```python
from build123d import *

# Parameters (mm, degrees)
SKETCH1_W                                       = 98.4125
SKETCH1_H                                       = 300
BOSS_EXTRUDE1_DEPTH                             = 0.79375
CHAMFER1_SIZE                                   = 0.79375
CUT_EXTRUDE1_DEPTH                              = 2.5875
FILLET1_R                                       = 3.5
CSK_FOR_M3_FLAT_HEAD_MACHINE_SCREW1_D           = 3.4
CSK_FOR_M3_FLAT_HEAD_MACHINE_SCREW1_DEPTH       = 7.596
CSK_FOR_M3_FLAT_HEAD_MACHINE_SCREW1_CSINK_D     = 6.3
CSK_FOR_M3_FLAT_HEAD_MACHINE_SCREW1_CSINK_ANGLE = 90
CSK_FOR_M3_FLAT_HEAD_MACHINE_SCREW1_TIP         = 1.021463052


with BuildPart() as part:
    # Sketch1 → Boss-Extrude1 (new body, symmetric)
    with BuildSketch(Plane.XY):
        Rectangle(SKETCH1_W, SKETCH1_H)
    extrude(amount=BOSS_EXTRUDE1_DEPTH, both=True)

    # Chamfer1
    chamfer1_edges = [part.edges().sort_by_distance(p)[0] for p in [
        (49.20625, 0, -0.79375),
        (-49.20625, 0, -0.79375),
    ]]
    chamfer(chamfer1_edges, length=CHAMFER1_SIZE)

    # Sketch2 → Cut-Extrude1 (cut, through all)
    with BuildSketch(Plane(origin=(0, 0, -0.79375), x_dir=(-1, 0, 0), z_dir=(0, 0, -1))):
        Polygon((28.868145751, 70.95), (0, 99.818145751), (-28.868145751, 70.95), align=None)
        Polygon((-38.4125, 72.719354249), (-38.4125, 138.230645751), (-5.656854249, 105.475), align=None)
        Polygon((28.868145751, 140), (-28.868145751, 140), (0, 111.131854249), align=None)
        Polygon((38.4125, 138.230645751), (38.4125, 72.719354249), (5.656854249, 105.475), align=None)
        with BuildLine():
            Line((10, 49.95), (35, 49.95))
            ThreePointArc((35, 49.95), (38, 52.95), (35, 55.95))
            Line((35, 55.95), (10, 55.95))
            ThreePointArc((10, 55.95), (7, 52.95), (10, 49.95))
        make_face()
        with BuildLine():
            Line((-35, 21.95), (-10, 21.95))
            ThreePointArc((-10, 21.95), (-7, 24.95), (-10, 27.95))
            Line((-10, 27.95), (-35, 27.95))
            ThreePointArc((-35, 27.95), (-38, 24.95), (-35, 21.95))
        make_face()
        with BuildLine():
            Line((-35, 55.95), (-10, 55.95))
            ThreePointArc((-10, 55.95), (-7, 52.95), (-10, 49.95))
            Line((-10, 49.95), (-35, 49.95))
            ThreePointArc((-35, 49.95), (-38, 52.95), (-35, 55.95))
        make_face()
        with BuildLine():
            Line((-35, 41.95), (-10, 41.95))
            ThreePointArc((-10, 41.95), (-7, 38.95), (-10, 35.95))
            Line((-10, 35.95), (-35, 35.95))
            ThreePointArc((-35, 35.95), (-38, 38.95), (-35, 41.95))
        make_face()
        with BuildLine():
            Line((10, 41.95), (35, 41.95))
            ThreePointArc((35, 41.95), (38, 38.95), (35, 35.95))
            Line((35, 35.95), (10, 35.95))
            ThreePointArc((10, 35.95), (7, 38.95), (10, 41.95))
        make_face()
        with BuildLine():
            Line((10, 27.95), (35, 27.95))
            ThreePointArc((35, 27.95), (38, 24.95), (35, 21.95))
            Line((35, 21.95), (10, 21.95))
            ThreePointArc((10, 21.95), (7, 24.95), (10, 27.95))
        make_face()
    extrude(amount=-CUT_EXTRUDE1_DEPTH, mode=Mode.SUBTRACT)

    # Fillet1
    fillet1_edges = [part.edges().sort_by_distance(p)[0] for p in [
        (38.4125, 72.719354249, 0),
        (38.4125, 138.230645751, 0),
        (5.656854249, 105.475, 0),
        (-38.4125, 138.230645751, 0),
        (-38.4125, 72.719354249, 0),
        (-5.656854249, 105.475, 0),
        (0, 99.818145751, 0),
        (-28.868145751, 70.95, 0),
        (28.868145751, 70.95, 0),
        (28.868145751, 140, 0),
        (-28.868145751, 140, 0),
        (0, 111.131854249, 0),
    ]]
    fillet(fillet1_edges, radius=FILLET1_R)

    # CSK for M3 Flat Head Machine Screw1
    with Locations(Plane.XY.offset(0.79375)):
        with Locations((-30, -145.225), (30, -145.225), (-30, 65.7), (30, 65.7), (30, 145.225), (-30, 145.225)):
            CounterSinkHole(CSK_FOR_M3_FLAT_HEAD_MACHINE_SCREW1_D / 2, CSK_FOR_M3_FLAT_HEAD_MACHINE_SCREW1_CSINK_D / 2, depth=CSK_FOR_M3_FLAT_HEAD_MACHINE_SCREW1_DEPTH, counter_sink_angle=CSK_FOR_M3_FLAT_HEAD_MACHINE_SCREW1_CSINK_ANGLE)
            with Locations((0, 0, -(CSK_FOR_M3_FLAT_HEAD_MACHINE_SCREW1_DEPTH + CSK_FOR_M3_FLAT_HEAD_MACHINE_SCREW1_TIP / 2))):  # 118° drill point
                Cone(0, CSK_FOR_M3_FLAT_HEAD_MACHINE_SCREW1_D / 2, CSK_FOR_M3_FLAT_HEAD_MACHINE_SCREW1_TIP, mode=Mode.SUBTRACT)


solid = part.part
```
CAD build for the part. Positions are in the model's coordinates, mm. A direction names the side the tool comes from. Coordinates: 2 decimals unless noted, no trailing zeros. Write each loop counter-clockwise with the first axis right and the second up, starting at its lowest first coordinate (ties: lowest second). Pieces come first, ordered by that corner, then holes.
(1) Drill centre lines: probe 1 along X at (y, z) = (65.7, -0.75); probe 2 along X at (y, z) = (110.5, 0.4); probe 3 along Y at (x, z) = (-2, 0.7). Where is each one in solid material? Low to high.
(2) Cut at A-A, the plane y = 52.95. List the corners of the cut face in (x, z).
(3) 3-axis set-ups, long thin cutter, end or side, ignore diameter. For faces 3 (the face through (-20.11, 119.93, -0.01)), 4 (the face through (-1, -31, -0.794)): which of +Z, -Z, +X, -X, +Y, -Y reach the whole face in a straight line?
(4) Cut at B-B, the plane y = 124. List the corners of the cut face in (x, z).
(5) Flat gauge pins, fed straight in: pin 1 (4 mm diameter, centred on x = -30, y = -145.225, fed in from +Z); pin 2 (0.8 mm diameter, centred on y = 107.5, z = -0.5, fed in from -X). Where does each tip first touch, or does it go through?
(6) Two-plate mould, pull along Y, no slides. Class faces 1 (the face through (12.54, 87.28, -0.01)), 2 (the face through (-1, -31, 0.794)): +Y half, -Y half, draft (parallel to the pull), parting line (faces both ways), or undercut.
(7) Cut at C-C, the plane z = -0.3. Count the separate pieces of the cut face and the enclosed holes in it, and give its area (3 significant figures).
Geometry says:
1. probe 1: x = -48.46 to -31.7, -28.3 to 28.3, 31.7 to 48.46
1. probe 2: x = -49.21 to -38.41, -10.68 to 10.68, 38.41 to 49.21
1. probe 3: y = -150 to 70.95, 97.74 to 113.21, 140 to 150
2. outline: (-49.21, 0) - (-48.41, -0.79) - (-38, -0.79) - (-38, 0.79) - (-49.21, 0.79) - close; (-7, -0.79) - (7, -0.79) - (7, 0.79) - (-7, 0.79) - close; (38, -0.79) - (48.41, -0.79) - (49.21, 0) - (49.21, 0.79) - (38, 0.79) - close
3. face 3: +Z, -Z
3. face 4: -Z, +X, -X, +Y, -Y
4. outline: (-49.21, 0) - (-48.41, -0.79) - (-38.41, -0.79) - (-38.41, 0.79) - (-49.21, 0.79) - close; (-24.18, -0.79) - (-12.87, -0.79) - (-12.87, 0.79) - (-24.18, 0.79) - close; (12.87, -0.79) - (24.18, -0.79) - (24.18, 0.79) - (12.87, 0.79) - close; (38.41, -0.79) - (48.41, -0.79) - (49.21, 0) - (49.21, 0.79) - (38.41, 0.79) - close
5. pin 1: stops at z = -0.36
5. pin 2: stops at x = -49.11
6. face 1: undercut
6. face 2: draft
7. separate pieces: 1
7. enclosed holes: 16
7. area: 24,500 mm2
